```python
from build123d import *

# Parameters (mm, degrees)
ESQUISSE1_R                  = 15
ESQUISSE1_R_2                = 2.5
BOSS_EXTRU_1_DEPTH           = 5
ENL_V_MAT_EXTRU_1_DEPTH      = 22.794494718
ENL_V_MAT_EXTRU_1_DEPTH_BACK = 22.794494718
ESQUISSE2_R                  = 1.5
ENL_V_START                  = -10
ENL_V_MAT_EXTRU_3_DEPTH      = 10
CONG_2_R                     = 0.5


with BuildPart() as part:
    # Esquisse1 → Boss.-Extru.1 (new body)
    with BuildSketch(Plane.XY):
        Circle(ESQUISSE1_R)
        Circle(ESQUISSE1_R_2, mode=Mode.SUBTRACT)
    extrude(amount=BOSS_EXTRU_1_DEPTH)

    # Esquisse2 → Enlèv. mat.-Extru.1 (cut, two sides: drawn at the far end of the back side and taken through both)
    with BuildSketch(Plane(origin=(0, 0, 0), x_dir=(1, 0, 0), z_dir=(0, 1, 0)).offset(-ENL_V_MAT_EXTRU_1_DEPTH_BACK)):
        with Locations(Location((-10, -2.5, 0), (0, 0, 270))):
            Circle(ESQUISSE2_R)
    extrude(amount=ENL_V_MAT_EXTRU_1_DEPTH + ENL_V_MAT_EXTRU_1_DEPTH_BACK, mode=Mode.SUBTRACT)

    # Esquisse3 → Enlèv. mat.-Extru.3 (cut)
    with BuildSketch(Plane.XY.offset(5).offset(ENL_V_START)):
        with BuildLine():
            Line((-14.924811557, 1.5), (-2.5, 1.5))
            Line((-2.5, 1.5), (-2, 1.5))
            ThreePointArc((-2, 1.5), (-2.5, 0), (-2, -1.5))
            Line((-2, -1.5), (-2.5, -1.5))
            Line((-2.5, -1.5), (-14.924811557, -1.5))
            ThreePointArc((-14.924811557, -1.5), (-15, 0), (-14.924811557, 1.5))
        make_face()
    extrude(amount=ENL_V_MAT_EXTRU_3_DEPTH, mode=Mode.SUBTRACT)

    # Congé2
    cong_2_edges = [part.edges().sort_by_distance(p)[0] for p in [
        (-2, 1.5, 2.5),
        (-2, -1.5, 2.5),
    ]]
    fillet(cong_2_edges, radius=CONG_2_R)


solid = part.part
```
Geometry: final body of the model. Coordinates: model frame, mm. A direction names the side the tool comes from. Give positions to 0.01 mm unless a question says otherwise; leave off trailing zeros. Loops run counter-clockwise (first coordinate to the right, second up) from the corner with the lowest first, then second, coordinate; pieces in that order, holes last. Notation, with made-up numbers: (57.5, 75) - (112.5, 75) arc R17 ccw to (112.5, 80) - close; hole circle Ø6 at (42, 50). An arc over 180 degrees is marked (long way). Answer as CSV lines item,"result". Start each with the question number.
(1) Pin query (flat end, axial travel): P1, Ø5, axis at x = 3, y = -8.5, coming from the -Z side; P2, Ø1.5, axis at x = -5.5, z = 3.5, coming from the -Y side; P3, Ø3, axis at x = 0, y = 0, coming from the -Z side; P4, Ø1.5, axis at x = -5.5, z = 3.5, coming from the +Y side. Return the tip coordinate at first contact, or that it passes through.
(2) Ray query, line 1 along Z through (x, y) = (-10, -7.5); line 2 along X through (y, z) = (8.5, 2.5); line 3 along X through (y, z) = (0, 3). Return the intervals inside material, ascending. Write a range as [from, to].
(3) Section query C-C (y = 8). Output: boundary loops of the cut face in (x, z).
(4) Section query B-B (z = 2.9). Output: boundary loops of the cut face in (x, y).
(5) Section query A-A (x = 0). Output: boundary loops of the cut face in (y, z).
(6) Section query D-D (x = -10.75). Output: boundary loops of the cut face in (y, z), and give its area (3 significant figures).
(7) Mould query, pull axis X, two halves, no side actions, for faces 1 (the face through (-8, -1.5, 2)), 2 (the face through (2.5, -0.1, 2.5)). Classes: +X half, -X half, draft (parallel to the pull), parting line (faces both ways), or undercut.
(8) Reachability of faces 3 (the face through (-9, 1.5, 1)), 4 (the face through (-8.513, -7.006, 2.305)) from +Z, -Z, +X, -X, +Y, -Y: full face, straight path, thin tool, end or side. Return the list, or none.
Worked answers:
1,P1,"stops at z = 0"
1,P2,"stops at y = -14.23"
1,P3,"passes through"
1,P4,"stops at y = 14.23"
2,line 1,"z = [0, 1], [4, 5]"
2,line 2,"x = [-12.36, -11.5], [-8.5, 12.36]"
2,line 3,"x = [2.5, 15]"
3,outline,"(-12.69, 0) - (12.69, 0) - (12.69, 5) - (-12.69, 5) - close; hole circle Ø3 at (-10, 2.5)"
4,outline,"(-14.92, -1.5) arc R15 ccw to (-11.45, -9.7) - (-11.45, -1.5) - close; (-14.92, 1.5) - (-11.45, 1.5) - (-11.45, 9.7) arc R15 ccw to start; (-8.55, -12.32) arc R15 ccw (long way) to (-8.55, 12.32) - (-8.55, 1.5) - (-2.24, 1.5) arc R0.5 ccw to (-1.86, 1.67) arc R2.5 cw (long way) to (-1.86, -1.67) arc R0.5 ccw to (-2.24, -1.5) - (-8.55, -1.5) - close"
5,outline,"(-15, 0) - (-2.5, 0) - (-2.5, 5) - (-15, 5) - close; (2.5, 0) - (15, 0) - (15, 5) - (2.5, 5) - close"
6,outline,"(-10.46, 0) - (-1.5, 0) - (-1.5, 1.2) - (-10.46, 1.2) - close; (-10.46, 3.8) - (-1.5, 3.8) - (-1.5, 5) - (-10.46, 5) - close; (1.5, 0) - (10.46, 0) - (10.46, 1.2) - (1.5, 1.2) - close; (1.5, 3.8) - (10.46, 3.8) - (10.46, 5) - (1.5, 5) - close"
6,area,"43.0 mm^2"
7,face 1,"draft"
7,face 2,"undercut"
8,face 3,"+Z, -Z, -X"
8,face 4,"+Y, -Y"
